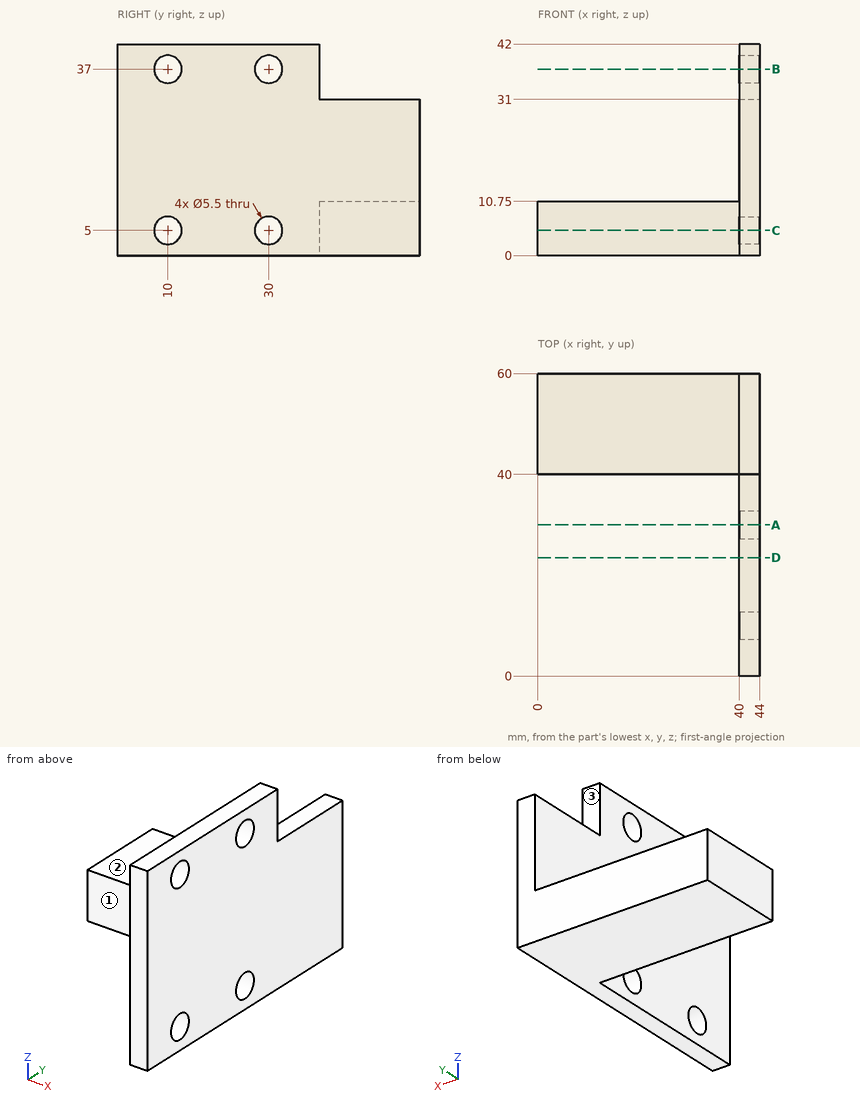
Geometry check sheet. Reference: drawing and pictorial views, mm from the part's lowest x, y, z. A direction names the side the tool comes from. Give positions to 0.01 mm unless a question says otherwise; leave off trailing zeros. Write each loop counter-clockwise with the first axis right and the second up, starting at its lowest first coordinate (ties: lowest second). Pieces come first, ordered by that corner, then holes.
Item 1: Gauge pin test, flat ends, axial feed: pin 1 (3 mm diameter, centred on y = 21, z = 18, fed in from -X); pin 2 (8 mm diameter, centred on x = 7, z = 13, fed in from -Y); pin 3 (3 mm diameter, centred on x = 41.5, y = 53, fed in from +Z). Record the tip position at first contact, or that the pin passes through.
Item 2: Scan lines: L1, parallel to Y at x = 41.75, z = 5; L2, parallel to Y at x = 41.6, z = 37; L3, parallel to X at y = 9.5, z = 13. Record each from-to range of solid material in increasing order.
Item 3: Cross-section at D-D (y = 23.5). Enter the section's corners in (x, z).
Item 4: Cross-section at C-C (z = 5). Enter the section's corners in (x, y).
Item 5: Cross-section at B-B (z = 37). Enter the section's corners in (x, y).
Item 6: Access from +Z, -Z, +X, -X, +Y, -Y to the whole of each face (thin tool, end or side, straight path). Record for the marked faces 1, 2 and 3.
Item 7: Cross-section at A-A (y = 30). Enter the section's corners in (x, z).
Report:
1. pin 1: stops at x = 40
1. pin 2: stops at y = 40
1. pin 3: stops at z = 31
2. L1: y = 0 to 7.25, 12.75 to 27.25, 32.75 to 60
2. L2: y = 0 to 7.25, 12.75 to 27.25, 32.75 to 40
2. L3: x = 40 to 44
3. outline: (40, 0) - (44, 0) - (44, 42) - (40, 42) - close
4. outline: (0, 40) - (40, 40) - (40, 32.75) - (44, 32.75) - (44, 60) - (0, 60) - close; (40, 0) - (44, 0) - (44, 7.25) - (40, 7.25) - close; (40, 12.75) - (44, 12.75) - (44, 27.25) - (40, 27.25) - close
5. outline: (40, 0) - (44, 0) - (44, 7.25) - (40, 7.25) - close; (40, 12.75) - (44, 12.75) - (44, 27.25) - (40, 27.25) - close; (40, 32.75) - (44, 32.75) - (44, 40) - (40, 40) - close
6. face 1: +Z, -Z, -X, -Y
6. face 2: +Z, -X, +Y, -Y
6. face 3: +Z, +X, -X, +Y
7. outline: (40, 0) - (44, 0) - (44, 2.25) - (40, 2.25) - close; (40, 7.75) - (44, 7.75) - (44, 34.25) - (40, 34.25) - close; (40, 39.75) - (44, 39.75) - (44, 42) - (40, 42) - close
